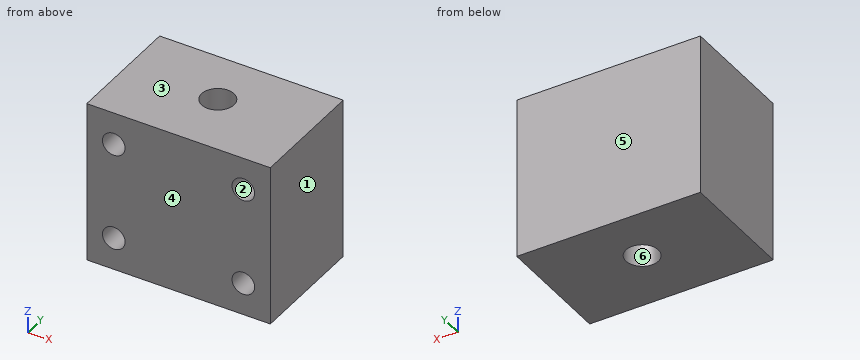
from build123d import *

# Parameters (mm, degrees)
SKETCH_1_W          = 34
SKETCH_1_H          = 30
EXTRUDE_1_DEPTH     = 22
SKETCH_2_R          = 3
CUT_EXTRUDE_1_DEPTH = 42.773197148
SKETCH_3_R          = 2.1
CUT_EXTRUDE_2_DEPTH = 10


with BuildPart() as part:
    # 草图1 → 凸台-拉伸1 (new body)
    with BuildSketch(Plane(origin=(0, 0, 0), x_dir=(1, 0, 0), z_dir=(0, 1, 0))):
        Rectangle(SKETCH_1_W, SKETCH_1_H)
    extrude(amount=EXTRUDE_1_DEPTH)

    # 草图2 → 切除-拉伸1 (cut, through all)
    with BuildSketch(Plane(origin=(2, 0, 15), x_dir=(-1, 0, 0), z_dir=(0, 0, -1))):
        with Locations((2, 11.846291658)):
            Circle(SKETCH_2_R)
    extrude(amount=CUT_EXTRUDE_1_DEPTH, mode=Mode.SUBTRACT)

    # 草图3 → 切除-拉伸2 (cut)
    with BuildSketch(Plane.XZ):
        with Locations(Location((12, 9, 0), (0, 0, 270))):
            Circle(SKETCH_3_R)
        with Locations(Location((12, -9, 0), (0, 0, 270))):
            Circle(SKETCH_3_R)
        with Locations(Location((-12, 9, 0), (0, 0, 270))):
            Circle(SKETCH_3_R)
        with Locations(Location((-12, -9, 0), (0, 0, 270))):
            Circle(SKETCH_3_R)
    extrude(amount=-CUT_EXTRUDE_2_DEPTH, mode=Mode.SUBTRACT)


solid = part.part
The model under review builds one solid part; all positions refer to its coordinate system, in mm. Face numbers are marked on the shaded views. A direction names the side the tool comes from. Round coordinates to 2 decimals unless told otherwise and drop trailing zeros. Loops run counter-clockwise (first coordinate to the right, second up) from the corner with the lowest first, then second, coordinate; pieces in that order, holes last. Notation, with made-up numbers: M 46.25,18 L 97.25,18 A30 cw 97.25,46 Z; hole C -36,37 d6. An arc over 180 degrees is marked long. Answer as CSV lines item,"result". Start each with the question number.
Item 1: Consider section C-C (x = 12). Write out the cut boundary in (y, z), then the cut area to 3 significant figures.
Item 2: Wall thickness on line 1 (X direction, y = 7.75, z = 9); line 2 (X direction, y = 11.75, z = -3.5); line 3 (Y direction, x = 0, z = -0.5): over which ranges is each line inside the solid? List them lowest first. Write a range as [from, to].
Item 3: Consider section D-D (z = -9). Write out the cut boundary in (x, y).
Item 4: For the marked faces 1 and 2, list the 3-axis set-ups (+Z, -Z, +X, -X, +Y, -Y) from which the entire face can be reached by the end or side of a thin tool; tool diameter is ignored.
Item 5: Consider section A-A (x = 0). Write out the cut boundary in (y, z), then the cut area to 3 significant figures.
Item 6: Insertion check: P1, Ø1.3, axis at x = -12.5, z = -9.5, coming from the -Y side; P2, Ø5.5, axis at x = 0, y = 11.85, coming from the +Z side. Each pin has a flat end and moves straight along its axis. Give the tip position at first contact, or say it passes through.
Item 7: Mouldability with a two-part tool opening along Y and no side actions: class the marked faces 3, 4, 5 and 6 as released by +Y, released by -Y, zero draft, split by the parting line, or undercut.
Item 8: Consider section B-B (y = 11.25). Write out the cut boundary in (x, z), then the cut area to 3 significant figures.
Answer:
1,outline,"M 0,-15 L 22,-15 L 22,15 L 0,15 L 0,11.1 L 10,11.1 L 10,6.9 L 0,6.9 L 0,-6.9 L 10,-6.9 L 10,-11.1 L 0,-11.1 Z"
1,area,"576 mm^2"
2,line 1,"x = [-17, -14.1], [-9.9, 9.9], [14.1, 17]"
2,line 2,"x = [-17, -3], [3, 17]"
2,line 3,"y = [0, 8.85], [14.85, 22]"
3,outline,"M -17,0 L -14.1,0 L -14.1,10 L -9.9,10 L -9.9,0 L 9.9,0 L 9.9,10 L 14.1,10 L 14.1,0 L 17,0 L 17,22 L -17,22 Z; hole C 0,11.85 d6"
4,face 1,"+Z, -Z, +X, +Y, -Y"
4,face 2,"-Y"
5,outline,"M 0,-15 L 8.85,-15 L 8.85,15 L 0,15 Z; M 14.85,-15 L 22,-15 L 22,15 L 14.85,15 Z"
5,area,"480 mm^2"
6,P1,"stops at y = 10"
6,P2,"passes through"
7,face 3,"zero draft"
7,face 4,"released by -Y"
7,face 5,"released by +Y"
7,face 6,"undercut"
8,outline,"M -17,-15 L -2.94,-15 L -2.94,15 L -17,15 Z; M 2.94,-15 L 17,-15 L 17,15 L 2.94,15 Z"
8,area,"844 mm^2"
